from build123d import *

# Parameters (mm, degrees)
BOSS_EXTRUDE1_DEPTH        = 13.97
SKETCH2_R                  = 2.54
CUT_EXTRUDE1_DEPTH         = 10.16
CUT_EXTRUDE3_START         = 6.35
SKETCH4_R                  = 1.27
CUT_EXTRUDE3_DEPTH         = 5.08
FILLET2_R                  = 1.27
CHAMFER2_SIZE              = 0.508
SCALE1_SCALE               = 1.5
F_50_0_07_DIAMETER_HOLE1_D = 1.778


with BuildPart() as part:
    # Sketch1 → Boss-Extrude1 (new body)
    with BuildSketch(Plane(origin=(0, 0, 0), x_dir=(1, 0, 0), z_dir=(0, 1, 0))):
        with BuildLine():
            Line((-5.08, 2.54), (-3.81, 2.54))
            Line((-3.81, 2.54), (-3.81, -2.54))
            Line((-3.81, -2.54), (-5.08, -2.54))
            Line((-5.08, -2.54), (-5.08, -5.08))
            Line((-5.08, -5.08), (0, -5.08))
            ThreePointArc((0, -5.08), (5.08, 0), (0, 5.08))
            Line((0, 5.08), (-5.08, 5.08))
            Line((-5.08, 5.08), (-5.08, 2.54))
        make_face()
    extrude(amount=BOSS_EXTRUDE1_DEPTH)

    # Sketch2 → Cut-Extrude1 (cut)
    with BuildSketch(Plane(origin=(0, 13.97, 0), x_dir=(1, 0, 0), z_dir=(0, 1, 0))):
        with Locations(Location((0, 0, 0), (0, 0, 270))):
            Circle(SKETCH2_R)
    extrude(amount=-CUT_EXTRUDE1_DEPTH, mode=Mode.SUBTRACT)

    # Sketch4 → Cut-Extrude3 (cut)
    with BuildSketch(Plane(origin=(0, 0, 0), x_dir=(0, 0, -1), z_dir=(1, 0, 0)).offset(CUT_EXTRUDE3_START)):
        with Locations((-3.556, 2.032)):
            Circle(SKETCH4_R)
        with Locations((3.556, 2.032)):
            Circle(SKETCH4_R)
        with Locations((-3.556, 11.938)):
            Circle(SKETCH4_R)
        with Locations((3.556, 11.938)):
            Circle(SKETCH4_R)
    extrude(amount=-CUT_EXTRUDE3_DEPTH, mode=Mode.SUBTRACT)

    # Fillet2
    fillet2_edges = [part.edges().sort_by_distance(p)[0] for p in [
        (-5.08, 6.985, -5.08),
        (-5.08, 6.985, 5.08),
    ]]
    fillet(fillet2_edges, radius=FILLET2_R)

    # Chamfer2
    chamfer2_edges = [part.edges().sort_by_distance(p)[0] for p in [
        (0, 13.97, -2.54),
    ]]
    chamfer(chamfer2_edges, length=CHAMFER2_SIZE)


with BuildPart() as part_1:
    # Scale1: scaled about (-0.295942874, 6.548984476, -4.0012e-05)
    add(part.part.scale(SCALE1_SCALE).moved(Location((0.147971437, -3.274492238, 2.0006e-05))))

    # #50 (0.07) Diameter Hole1 (through all)
    with Locations(Plane(origin=(2.052964344, 0, 0), x_dir=(0, 0, -1), z_dir=(1, 0, 0))):
        with Locations((-5.334026182, -0.226506275), (5.333973818, -0.226506275), (5.333973818, 14.632493725), (-5.334026182, 14.632493725)):
            Hole(F_50_0_07_DIAMETER_HOLE1_D / 2)


solid = part_1.part
Verification items for the finished model (mm, model axes). A direction names the side the tool comes from. Give positions to 0.01 mm unless a question says otherwise; leave off trailing zeros. Loops run counter-clockwise (first coordinate to the right, second up) from the corner with the lowest first, then second, coordinate; pieces in that order, holes last. Notation, with made-up numbers: (-32, 62) - (23, 62) arc R34 cw to (23, 94) - close; hole circle Ø11 at (-19.5, 51.5). An arc over 180 degrees is marked (long way). Write item = value, one per line. Start each with the question number.
Q1. Cross-section at D-D, the plane y = 1.25. Enter the section's corners in (x, z) (3 decimals), and give its area (3 significant figures).
Q2. Mould release check, pull along X, two halves, no side actions. Record for faces 1 (the face through (7.766, 7.056, 0.168)), 2 (the face through (-7.472, 7, -5)), 3 (the face through (-2.776, 14.672, 4.446)), 4 (the face through (3.926, 9.781, -0.496)): released by +X, released by -X, zero draft, split by the parting line, or undercut.
Q3. Tool access check on faces 5 (the face through (-7, 7, -3.81)), 6 (the face through (2.053, 1, 5)), 7 (the face through (-6.929, 7.35, 7.047)). Record the directions out of +Z, -Z, +X, -X, +Y, -Y that give a thin tool (end or side, any length) a straight path to the whole face; none if there is none.
Q4. Cross-section at A-A, the plane x = -6. Enter the section's corners in (y, z).
Q5. Cross-section at B-B, the plane y = 11.25. Enter the section's corners in (x, z) (3 decimals), and give its area (3 significant figures).
Q6. Thickness scan on line 1 (Y direction, x = -3.5, z = 0); line 2 (Z direction, x = 0.5, y = 11.75); line 3 (X direction, y = 4, z = -3.5). Record the ranges inside material, lowest first.
Q7. Depth check by flat-ended pin: P1, Ø2.5, axis at y = -0.23, z = -5.33, coming from the -X side; P2, Ø1.9, axis at y = 15, z = -6, coming from the +X side; P3, Ø1, axis at x = -6.5, y = 9.5, coming from the -Z side; P4, Ø4, axis at y = 0, z = 5, coming from the +X side. Enter the tip coordinate at first touch or a pass-through.
Q8. Cross-section at C-C, the plane x = 6.25. Enter the section's corners in (y, z) (1 decimal).
Answer key:
q1.outline = (-7.472, -5.715) arc R1.905 ccw to (-5.567, -7.62) - (0.148, -7.62) arc R7.62 ccw to (4.062, -6.538) - (2.053, -6.538) - (2.053, -4.13) - (6.552, -4.13) arc R7.62 ccw to (6.552, 4.13) - (2.053, 4.13) - (2.053, 6.538) - (4.062, 6.538) arc R7.62 ccw to (0.148, 7.62) - (-5.567, 7.62) arc R1.905 ccw to (-7.472, 5.715) - (-7.472, 3.81) - (-5.567, 3.81) - (-5.567, -3.81) - (-7.472, -3.81) - close
q1.area = 175 mm^2
q2.face_1 = released by +X
q2.face_2 = released by -X
q2.face_3 = zero draft
q2.face_4 = undercut
q3.face_5 = -X, +Y, -Y
q3.face_6 = +X
q3.face_7 = +Z, -X, +Y, -Y
q4.outline = (-3.27, -7.57) - (17.68, -7.57) - (17.68, -3.81) - (-3.27, -3.81) - close; (-3.27, 3.81) - (17.68, 3.81) - (17.68, 7.57) - (-3.27, 7.57) - close; hole circle Ø1.78 at (-0.23, -5.33); hole circle Ø1.78 at (-0.23, 5.33); hole circle Ø1.78 at (14.63, -5.33); hole circle Ø1.78 at (14.63, 5.33)
q5.outline = (-7.472, -5.715) arc R1.905 ccw to (-5.567, -7.62) - (0.148, -7.62) arc R7.62 ccw to (0.148, 7.62) - (-5.567, 7.62) arc R1.905 ccw to (-7.472, 5.715) - (-7.472, 3.81) - (-5.567, 3.81) - (-5.567, -3.81) - (-7.472, -3.81) - close; hole circle Ø7.62 at (0.148, 0)
q5.area = 146 mm^2
q6.line_1 = -3.27 to 2.44
q6.line_2 = -7.61 to -3.79, 3.79 to 7.61
q6.line_3 = -5.57 to -1.36, 1.65 to 6.92
q7.P1 = -7.47
q7.P2 = 2.05
q7.P3 = -7.57
q7.P4 = 7.15
q8.outline = (-3.3, -4.6) - (-2, -4.6) arc R1.9 cw to (1.5, -4.6) - (12.9, -4.6) arc R1.9 cw to (16.4, -4.6) - (17.7, -4.6) - (17.7, 4.6) - (16.4, 4.6) arc R1.9 cw to (12.9, 4.6) - (1.5, 4.6) arc R1.9 cw to (-2, 4.6) - (-3.3, 4.6) - close
